Work out the finished part from the listing and answer in its coordinate system (mm). Round coordinates to 2 decimals unless told otherwise and drop trailing zeros. Order: outer loops, then holes, each group sorted by start corner. A loop starts at its lowest first (then second) coordinate and runs counter-clockwise, first axis right, second up. Notation, with made-up numbers: (89.5, 61.25) - (103.5, 61.25) arc R17 cw to (103.5, 91.25) - close; hole circle Ø2 at (49, 79.25). An arc over 180 degrees is marked (long way). Answer in a Markdown table with one row per item.
from build123d import *

# Parameters (mm, degrees)
CROQUIS1_R              = 58
CROQUIS1_R_2            = 7
CROQUIS1_R_3            = 9
SALIENTE_EXTRUIR1_DEPTH = 10


with BuildPart() as part:
    # Croquis1 → Saliente-Extruir1 (new body)
    # profile 1 of 3: a face of its own
    with BuildSketch(Plane.XY):
        Circle(CROQUIS1_R)
        with Locations((-22.5, 38.97114317)):
            Circle(CROQUIS1_R_2, mode=Mode.SUBTRACT)
        with Locations((-38.97114317, 22.5)):
            Circle(CROQUIS1_R_2, mode=Mode.SUBTRACT)
        with Locations((-45, 0)):
            Circle(CROQUIS1_R_2, mode=Mode.SUBTRACT)
        with Locations((-38.97114317, -22.5)):
            Circle(CROQUIS1_R_2, mode=Mode.SUBTRACT)
        with Locations((-22.5, -38.97114317)):
            Circle(CROQUIS1_R_2, mode=Mode.SUBTRACT)
        with Locations((0, -45)):
            Circle(CROQUIS1_R_2, mode=Mode.SUBTRACT)
        with Locations((22.5, -38.97114317)):
            Circle(CROQUIS1_R_2, mode=Mode.SUBTRACT)
        with Locations((38.97114317, -22.5)):
            Circle(CROQUIS1_R_2, mode=Mode.SUBTRACT)
        with Locations((45, 0)):
            Circle(CROQUIS1_R_2, mode=Mode.SUBTRACT)
        with Locations((38.97114317, 22.5)):
            Circle(CROQUIS1_R_2, mode=Mode.SUBTRACT)
        with Locations((22.5, 38.97114317)):
            Circle(CROQUIS1_R_2, mode=Mode.SUBTRACT)
        with Locations((0, 45)):
            Circle(CROQUIS1_R_2, mode=Mode.SUBTRACT)
        with BuildLine():
            Line((5, 25), (5, 0))
            ThreePointArc((5, 0), (11, -6), (17, 0))
            ThreePointArc((17, 0), (25, 8), (33, 0))
            ThreePointArc((33, 0), (0, -33), (-33, 0))
            ThreePointArc((-33, 0), (-25, 8), (-17, 0))
            ThreePointArc((-17, 0), (-11, -6), (-5, 0))
            Line((-5, 0), (-5, 25))
            ThreePointArc((-5, 25), (0, 30), (5, 25))
        make_face(mode=Mode.SUBTRACT)
    # profile 2 of 3: a face of its own
    with BuildSketch(Plane.XY):
        with BuildLine():
            Line((1.58e-07, -58), (66, -58))
            ThreePointArc((66, -58), (80.964085993, -41.962632957), (63.930233382, -28.143484051))
            ThreePointArc((63.930233382, -28.143484051), (56.702087905, -25.367174857), (55.211041749, -17.769098711))
            ThreePointArc((55.211041749, -17.769098711), (34.156934021, -46.87540782), (1.58e-07, -58))
        make_face()
        with Locations((66, -43)):
            Circle(CROQUIS1_R_3, mode=Mode.SUBTRACT)
    # profile 3 of 3: a face of its own
    with BuildSketch(Plane.XY):
        with BuildLine():
            Line((-66, -58), (1.58e-07, -58))
            ThreePointArc((1.58e-07, -58), (-34.156933894, -46.875407913), (-55.211041749, -17.769098711))
            ThreePointArc((-55.211041749, -17.769098711), (-56.702087905, -25.367174857), (-63.930233382, -28.143484051))
            ThreePointArc((-63.930233382, -28.143484051), (-80.964085993, -41.962632957), (-66, -58))
        make_face()
        with Locations((-66, -43)):
            Circle(CROQUIS1_R_3, mode=Mode.SUBTRACT)
    extrude(amount=SALIENTE_EXTRUIR1_DEPTH)


solid = part.part
1) Find section A-A, the plane x = 25. Give the vertices of the cut face in (y, z).
Filled in:
| item | result |
|---|---|
| outline | (-58, 0) - (-45.51, 0) - (-45.51, 10) - (-58, 10) - close; (-32.43, 0) - (-21.54, 0) - (-21.54, 10) - (-32.43, 10) - close; (8, 0) - (32.43, 0) - (32.43, 10) - (8, 10) - close; (45.51, 0) - (52.34, 0) - (52.34, 10) - (45.51, 10) - close |
2) Find section D-D, the plane y = 48. Give the vertices of the cut face in (x, z), then the cut area to 3 significant figures.
Filled in:
| item | result |
|---|---|
| outline | (-32.56, 0) - (-6.32, 0) - (-6.32, 10) - (-32.56, 10) - close; (6.32, 0) - (32.56, 0) - (32.56, 10) - (6.32, 10) - close |
| area | 525 mm^2 |
3) Find section B-B, the plane z = 8. Give the number of separate pieces and of enclosed holes in the cut face, then the cut area to 3 significant figures.
Filled in:
| item | result |
|---|---|
| separate pieces | 1 |
| enclosed holes | 15 |
| area | 8,680 mm^2 |
4) Find the intervals of material crossed by probe 1 along Y at (x, z) = (0, 6.75); probe 2 along X at (y, z) = (35, 7); probe 3 along Y at (x, z) = (45, 6.75), in increasing order. Write a range as from..to.
Filled in:
| item | result |
|---|---|
| probe 1 | y = -58..-52, -38..-33, 30..38, 52..58 |
| probe 2 | x = -46.25..-28.26, -16.74..16.74, 28.26..46.25 |
| probe 3 | y = -58..-26.06, -18.94..-7, 7..18.94, 26.06..36.59 |
5) Find section C-C, the plane x = -11. Give the vertices of the cut face in (y, z), then the cut area to 3 significant figures.
Filled in:
| item | result |
|---|---|
| outline | (-58, 0) - (-31.11, 0) - (-31.11, 10) - (-58, 10) - close; (-6, 0) - (56.95, 0) - (56.95, 10) - (-6, 10) - close |
| area | 898 mm^2 |
6) The mould has two halves that part along Y. Classify faces 1 (the face through (16.87, 0.81, 0)), 2 (the face through (-1, -58, 5)), 3 (the face through (56.776, -25.453, 4.93)): released by +Y, released by -Y, zero draft, split by the parting line, or undercut.
Filled in:
| item | result |
|---|---|
| face 1 | zero draft |
| face 2 | released by -Y |
| face 3 | undercut |
7) Each of these flat-tipped pins is pushed along its axis until it touches: pin 1 (5 mm diameter, centred on y = 17.5, z = 3.5, fed in from -X); pin 2 (1.5 mm diameter, centred on y = 8, z = 5.5, fed in from +X). Where does it stop, or does it pass through?
Filled in:
| item | result |
|---|---|
| pin 1 | stops at x = -56.03 |
| pin 2 | stops at x = 57.55 |
